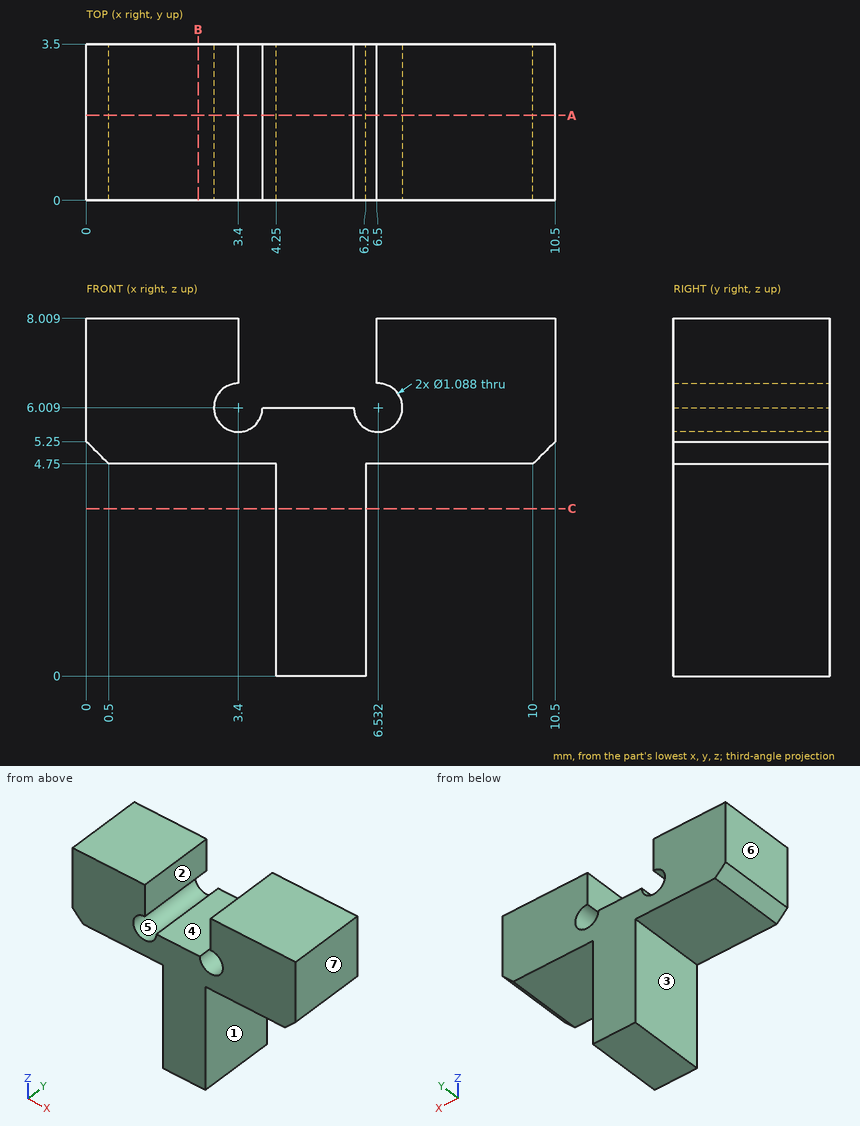
Geometry: see drawing. Coordinates: mm, zero at the bounding-box minimum. A direction names the side the tool comes from. Give positions to 0.01 mm unless a question says otherwise; leave off trailing zeros. Write each loop counter-clockwise with the first axis right and the second up, starting at its lowest first coordinate (ties: lowest second). Pieces come first, ordered by that corner, then holes. Notation, with made-up numbers: M 11.25,-4.5 L 32.25,-4.5 A26 cw 32.25,30.5 Z; hole C 76,1.5 d3. An arc over 180 degrees is marked long. Answer in a Markdown table with one row per item. Add a question column.
(1) First-contact query: pin 1 (1.8 mm diameter, centred on x = 8, y = 1.5, fed in from -Z); pin 2 (1.8 mm diameter, centred on y = 2, z = 1.5, fed in from +X); pin 3 (1.5 mm diameter, centred on y = 1.5, z = 3, fed in from -X); pin 4 (0.9 mm diameter, centred on x = 3.4, z = 6.01, fed in from +Y). Flat tips, straight axial feed; report the tip coordinate or a pass-through.
(2) Mould query, pull axis X, two halves, no side actions, for the marked faces 4, 5, 6 and 7. Classes: +X half, -X half, draft (parallel to the pull), parting line (faces both ways), or undercut.
(3) Reachability of the marked faces 1, 2 and 3 from +Z, -Z, +X, -X, +Y, -Y: full face, straight path, thin tool, end or side. Return the list, or none.
(4) Section A-A on y = 1.9. Return loops of the section in (x, z).
(5) Ray query, line 1 (X direction, y = 2.2, z = 7); line 2 (Z direction, x = 4.5, y = 0.85); line 3 (X direction, y = 2.55, z = 1). Return the intervals inside material, ascending.
(6) Section B-B on x = 2.5. Return loops of the section in (y, z), and give its area (3 significant figures).
(7) Section C-C on z = 3.75. Return loops of the section in (x, y).
Result set:
| question | item | result |
|---|---|---|
| 1 | pin 1 | stops at z = 4.75 |
| 1 | pin 2 | stops at x = 6.25 |
| 1 | pin 3 | stops at x = 4.25 |
| 1 | pin 4 | passes through |
| 2 | face 4 | undercut |
| 2 | face 5 | undercut |
| 2 | face 6 | -X half |
| 2 | face 7 | +X half |
| 3 | face 1 | -Z, +X, +Y, -Y |
| 3 | face 2 | +Z, +Y, -Y |
| 3 | face 3 | -Z, -X, +Y, -Y |
| 4 | outline | M 0,5.25 L 0.5,4.75 L 4.25,4.75 L 4.25,0 L 6.25,0 L 6.25,4.75 L 10,4.75 L 10.5,5.25 L 10.5,8.01 L 6.5,8.01 L 6.5,6.55 A0.54 cw long 5.99,6.01 L 3.94,6.01 A0.54 cw long 3.4,6.55 L 3.4,8.01 L 0,8.01 Z |
| 5 | line 1 | x = 0 to 3.4, 6.5 to 10.5 |
| 5 | line 2 | z = 0 to 6.01 |
| 5 | line 3 | x = 4.25 to 6.25 |
| 6 | outline | M 0,4.75 L 3.5,4.75 L 3.5,8.01 L 0,8.01 Z |
| 6 | area | 11.4 mm^2 |
| 7 | outline | M 4.25,0 L 6.25,0 L 6.25,3.5 L 4.25,3.5 Z |
